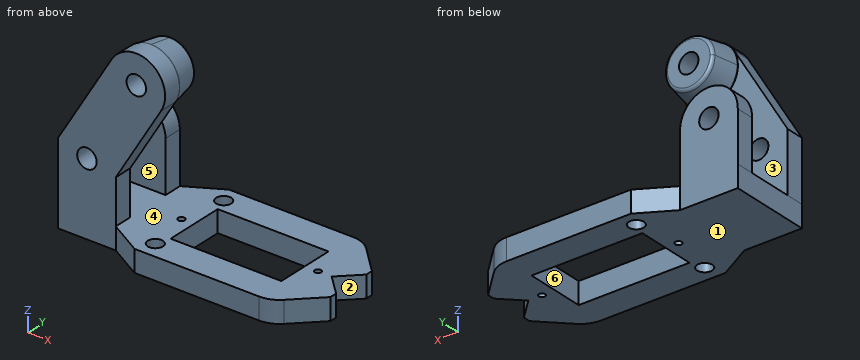
Solid Edge part; units mm, degrees
sketch "Sketch1" plane through (0, 0, 0) normal (0, 0, -1) x (-1, 0, 0)
  line L0 (-47.0429, 25.1351) -> (-19.0272, 25.1351)
  line L1 (-12.0091, 21.1302) -> (-19.0272, 25.1351)
  line L2 (-12.0091, 21.1302) -> (-0.0646, 21.1302)
  line L3 (-0.0646, 21.1302) -> (-0.0646, 12.6221)
  line L4 (-0.0646, 4.114) -> (-0.0646, 12.6221)
  line L5 (-12.0091, 4.114) -> (-0.0646, 4.114)
  line L6 (-12.0091, 4.114) -> (-19.0272, 0.1091)
  line L7 (-47.0429, 0.1091) -> (-19.0272, 0.1091)
  line L8 (-47.0429, 0.1091) -> (-54.082, 7.1192)
  line L9 (-54.082, 7.1192) -> (-54.082, 8.6266)
  line L10 (-54.082, 8.6266) -> (-50.0417, 12.6221)
  line L11 (-54.082, 16.6176) -> (-50.0417, 12.6221)
  line L12 (-54.082, 18.1251) -> (-54.082, 16.6176)
  line L13 (-47.0429, 25.1351) -> (-54.082, 18.1251)
extrude "Protrusion1" add sketch "Sketch1" against normal blind 4.5
sketch "Sketch2" plane through (6.0368, 4.114, 2.25) normal (0, -1, 0) x (1, 0, 0)
  line L0 (-5.9723, 2.25) -> (-5.9723, 14.6813)
  line L1 (-5.9723, 14.6813) -> (5.1048, 33.2011)
  arc A0 (5.1048, 33.2011) -> (15.3315, 27.0843) centre (10.2182, 30.1427) cw
  line L2 (5.9723, 11.4366) -> (15.3315, 27.0843)
  line L3 (5.9723, 2.25) -> (5.9723, 11.4366)
  line L4 (-5.9723, 2.25) -> (5.9723, 2.25)
extrude "Ajout_matière_2" add sketch "Sketch2" against normal blind 3.81
sketch "Sketch3" plane through (6.0368, 21.1302, 2.25) normal (0, 1, 0) x (-1, 0, 0)
  line L0 (5.9723, 12.5868) -> (5.9723, 2.25)
  line L1 (-5.9723, 2.25) -> (5.9723, 2.25)
  line L2 (-5.9723, 12.8853) -> (-5.9723, 2.25)
  arc A0 (5.9723, 12.5868) -> (-5.9723, 12.8853) centre (0, 12.7361) ccw
extrude "Ajout_matière_3" add sketch "Sketch3" against normal blind 3.81
sketch "Sketch4" plane through (6.0368, 21.1302, 2.25) normal (0, 1, 0) x (-1, 0, 0)
  circle A0 centre (0, 12.8992) radius 2.0092
extrude "Cutout1" cut sketch "Sketch4" against normal through all
sketch "Sketch5" plane through (11.1416, 7.924, 35.4511) normal (-0.513309, 0, -0.8582039) x (0, -1, 0)
  line L0 (-0.1674, -5.9582) -> (-5.3937, -5.9582)
  line L1 (-0.1674, -5.9582) -> (0, -5.9582)
sketch "Sketch6" plane through (16.255, 7.924, 32.3927) normal (0, 1, 0) x (-1, 0, 0)
  circle A0 centre (0, 0) radius 5.9106
sketch "Sketch7" plane through (11.1389, 13.385, 21.4255) normal (0, 1, 0) x (0, 0, 1)
  circle A0 centre (10.9673, 5.1161) radius 4.9379
sweep "Ajout_matière_par_balayage_4" add profiles "Sketch6", "Sketch7" path "Sketch5"
sketch "Sketch8" plane through (16.255, 13.385, 32.3927) normal (0, 1, 0) x (-1, 0, 0)
  circle A0 centre (0, 0) radius 2.0106
extrude "Cutout2" cut sketch "Sketch8" against normal through all
sketch "Sketch9" plane through (27.0733, 12.6221, 4.5) normal (0, 0, 1) x (-1, 0, 0)
  circle A0 centre (8.1244, -0.0193) radius 0.6833
  circle A1 centre (-20.1211, -0.0193) radius 0.6456
  circle A2 centre (6.4635, 9.0435) radius 1.5652
  circle A3 centre (6.4635, -9.0821) radius 1.5652
  line L0 (-17.4191, 6.2241) -> (5.5043, 6.2241)
  line L1 (5.5043, 6.2241) -> (5.5043, -6.2627)
  line L2 (5.5043, -6.2627) -> (-17.4191, -6.2627)
  line L3 (-17.4191, -6.2627) -> (-17.4191, 6.2241)
  dimension "D1" = 6.4635
extrude "Cutout3" cut sketch "Sketch9" against normal through all
fillet "Congé_2" radius 5.5563 2 edges at (47.0429, 25.1351, 2.25) (47.0429, 0.1091, 2.25)
fillet "Congé_3" radius 0.635 1 edges at (21.1929, 13.385, 32.3927)
properties part number "AC_1.09"
Model file for the job. Use its own axes, mm. Face numbers are marked on the shaded views. A direction names the side the tool comes from. Give positions to 0.01 mm unless a question says otherwise; leave off trailing zeros. Order: outer loops, then holes, each group sorted by start corner. A loop starts at its lowest first (then second) coordinate and runs counter-clockwise, first axis right, second up. Notation, with made-up numbers: (-10, -9) - (4, -9) arc R14 ccw to (4, -4) - close; hole circle Ø1 at (25.5, 25). An arc over 180 degrees is marked (long way). One line per item, written item: value.
Item 1: Tool access for the marked faces 4, 5 and 6: list every direction of +Z, -Z, +X, -X, +Y, -Y with a clear straight run to the whole face (end or side of a thin tool).
Response values:
face 4: +X
face 5: +Z, +X, -X
face 6: +Z, -Z
Item 2: Pin check, flat tips, straight feed: pin 1 Ø4.5 at (x, z) = (6.04, 15.15) entering from +Y; pin 2 Ø4 at (x, y) = (13.5, 17.5) entering from +Z; pin 3 Ø1 at (x, y) = (42.5, 4.5) entering from -Z; pin 4 Ø9.5 at (x, z) = (14, 32.5) entering from +Y (3 decimals). Stop position of each tip, or through.
Response values:
pin 1: y = 21.13
pin 2: z = 17.4
pin 3: z = 0
pin 4: y = 13.385
Item 3: Slice it at A-A (x = 39). List the corners of the cut face in (y, z), then the cut area to 3 significant figures.
Response values:
outline: (0.11, 0) - (6.4, 0) - (6.4, 4.5) - (0.11, 4.5) - close; (18.88, 0) - (25.14, 0) - (25.14, 4.5) - (18.88, 4.5) - close
area: 56.4 mm2
Item 4: Wall check: line 1 (Y direction, x = 9, z = 13.5); line 2 (X direction, y = 7.5, z = 5); line 3 (Y direction, x = 12, z = 18). Give the ranges that are in metal, low to high.
Response values:
line 1: 4.11 to 7.92, 17.32 to 21.13
line 2: 0.06 to 12.01
line 3: 4.11 to 7.92
Item 5: Slice it at D-D (z = 23.5). List the corners of the cut face in (x, y), then the cut area to 3 significant figures.
Response values:
outline: (3.99, 4.11) - (17.88, 4.11) - (17.88, 7.92) - (3.99, 7.92) - close
area: 52.9 mm2
Item 6: Slice it at B-B (y = 16). List the corners of the cut face in (x, z).
Response values:
outline: (0.06, 0) - (21.57, 0) - (21.57, 4.5) - (0.06, 4.5) - close; (44.49, 0) - (53.46, 0) - (53.46, 4.5) - (44.49, 4.5) - close
Item 7: Two-plate mould, pull along Z, no slides. Class the marked faces 1, 2 and 3: released by +Z, released by -Z, zero draft, split by the parting line, or undercut.
Response values:
face 1: released by -Z
face 2: zero draft
face 3: undercut
